Input: dimensioned drawing with shaded views. Units: mm. Origin: part minimum x, y, z. Give positions to 0.01 mm unless a question says otherwise; leave off trailing zeros. Order: outer loops, then holes, each group sorted by start corner. A loop starts at its lowest first (then second) coordinate and runs counter-clockwise, first axis right, second up. Notation, with made-up numbers: M -1,0.25 L 58,0.25 A9 ccw 58,17.25 Z; hole C -10,33 d10. An arc over 180 degrees is marked long. Answer in a Markdown table with one row per item. Add a question column.
(1) Mould query, pull axis Z, two halves, no side actions, for the marked faces 1 and 2. Classes: pulls with the +Z half, pulls with the -Z half, needs draft (parallel to the pull), parting line crosses it, or undercut.
(2) Pin query (flat end, axial travel): P1, Ø14.5, axis at x = 48.45, z = 39.22, coming from the -Y side; P2, Ø3, axis at y = 4, z = 28.5, coming from the -X side; P3, Ø4.5, axis at x = 6.69, z = 71.75, coming from the +Y side (1 decimal); P4, Ø3, axis at x = 90.21, z = 71.75, coming from the +Y side (1 decimal). Return the tip coordinate at first contact, or that it passes through.
(3) Section query A-A, the plane y = 5.25. Return loops of the section in (x, z) (1 decimal).
(4) Material intervals for line 1 along X through (y, z) = (4.25, 40.5) (1 decimal); line 2 along Z through (x, y) = (85, 5.5) (1 decimal); line 3 along X through (y, z) = (6.5, 39), sorted ascending.
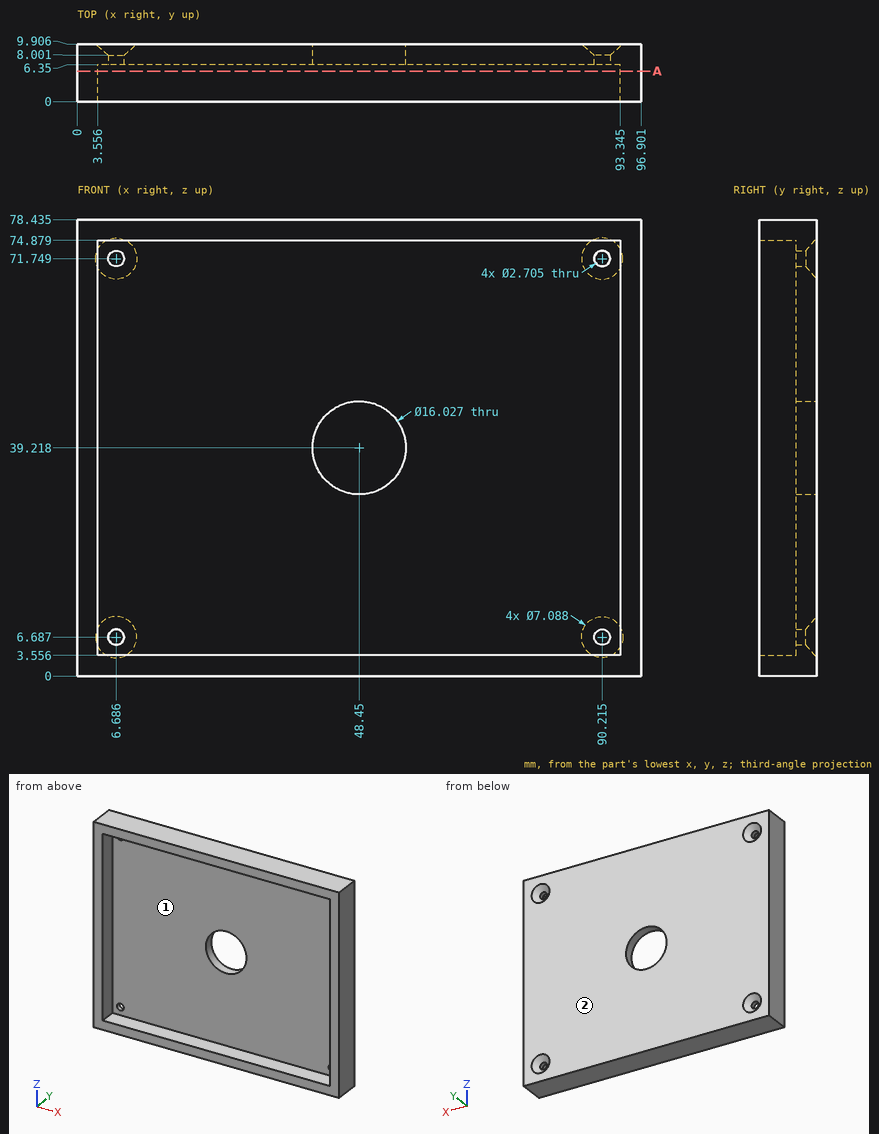
Values follow:
| question | item | result |
|---|---|---|
| 1 | face 1 | undercut |
| 1 | face 2 | needs draft |
| 2 | P1 | passes through |
| 2 | P2 | stops at x = 0 |
| 2 | P3 | stops at y = 8.8 |
| 2 | P4 | stops at y = 8.1 |
| 3 | outline | M 0,0 L 96.9,0 L 96.9,78.4 L 0,78.4 Z; hole M 3.6,3.6 L 93.3,3.6 L 93.3,74.9 L 3.6,74.9 Z |
| 4 | line 1 | x = 0 to 3.6, 93.3 to 96.9 |
| 4 | line 2 | z = 0 to 3.6, 74.9 to 78.4 |
| 4 | line 3 | x = 0 to 40.44, 56.46 to 96.9 |
